Build history of the part. All positions in model axes, mm. Round coordinates to 2 decimals unless told otherwise and drop trailing zeros. Write each loop counter-clockwise with the first axis right and the second up, starting at its lowest first coordinate (ties: lowest second). Pieces come first, ordered by that corner, then holes.
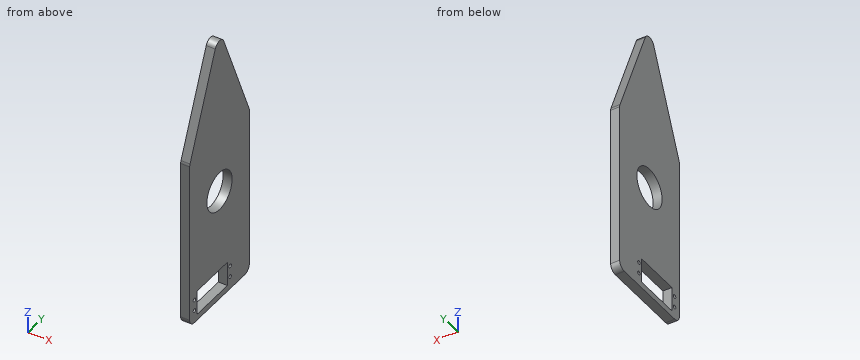
from build123d import *

# Parameters (mm, degrees)
SKETCH1_R                             = 17.4625
BOSS_EXTRUDE2_DEPTH                   = 4.0005
FILLET1_R                             = 6.35
TAP_DRILL_FOR_M4X0_7_TAP1_D           = 3.3
TAP_DRILL_FOR_M4X0_7_TAP1_CSINK_D     = 3.35
TAP_DRILL_FOR_M4X0_7_TAP1_CSINK_ANGLE = 90
SKETCH5_W                             = 42
SKETCH5_H                             = 22
CUT_EXTRUDE1_DEPTH                    = 148.97697313


with BuildPart() as part:
    # Sketch1 → Boss-Extrude2 (new, symmetric)
    with BuildSketch(Plane.YZ):
        Polygon((-41.275, 50.8), (-41.275, -101.6), (41.275, -101.6), (41.275, 50.8), (0, 152.4), align=None)
        with Locations(Location((0, 0, 0), (0, 0, 270))):
            Circle(SKETCH1_R, mode=Mode.SUBTRACT)
    extrude(amount=BOSS_EXTRUDE2_DEPTH, both=True)

    # Fillet1
    fillet1_edges = [part.edges().sort_by_distance(p)[0] for p in [
        (0, 0, 152.4),
        (0, 41.275, 50.8),
        (0, 41.275, -101.6),
        (0, -41.275, -101.6),
        (0, -41.275, 50.8),
    ]]
    fillet(fillet1_edges, radius=FILLET1_R)

    # Tap Drill for M4x0.7 Tap1 (through all)
    with Locations(Plane.YZ.offset(4.0005)):
        with Locations((-34.75, -80.25), (-34.75, -90.25), (14.75, -80.25), (14.75, -90.25)):
            CounterSinkHole(TAP_DRILL_FOR_M4X0_7_TAP1_D / 2, TAP_DRILL_FOR_M4X0_7_TAP1_CSINK_D / 2, counter_sink_angle=TAP_DRILL_FOR_M4X0_7_TAP1_CSINK_ANGLE)

    # Sketch5 → Cut-Extrude1 (cut, through all)
    with BuildSketch(Plane.YZ.offset(4.0005)):
        with Locations((-10, -85.25)):
            Rectangle(SKETCH5_W, SKETCH5_H)
    extrude(amount=-CUT_EXTRUDE1_DEPTH, mode=Mode.SUBTRACT)


solid = part.part
1) Wall check: L1, parallel to Y at x = 2.5, z = -80.25 (3 decimals); L2, parallel to Z at x = -3.25, y = -0.5; L3, parallel to Z at x = -2, y = 5. Give the ranges that are in metal, low to high.
Results:
L1: y = -41.275 to -36.4, -33.1 to -31, 11 to 13.1, 16.4 to 41.275
L2: z = -101.6 to -96.25, -74.25 to -17.46, 17.46 to 141.86
L3: z = -101.6 to -96.25, -74.25 to -16.73, 16.73 to 139.44
2) Slice it at A-A (x = -2.5). Count the separate pieces of the cut face and the enclosed holes in it, plus the area to 3 significant figures.
Results:
separate pieces: 1
enclosed holes: 6
area: 14,800 mm2
3) Pin check, flat tips, straight feed: pin 1 Ø1 at (x, y) = (-1, 31.5) entering from +Z; pin 2 Ø4 at (x, y) = (-0.5, -19.5) entering from +Z; pin 3 Ø2.5 at (y, z) = (-34.75, -90.25) entering from -X; pin 4 Ø2 at (x, y) = (1, -4) entering from +Z. Stop position of each tip, or through.
Results:
pin 1: stops at z = 76.09
pin 2: stops at z = 109.32
pin 3: passes through
pin 4: stops at z = 141.13
4) Slice it at B-B (z = 0). Write the cut outline in (x, y) (1 decimal).
Results:
outline: (-4, -41.3) - (4, -41.3) - (4, -17.5) - (-4, -17.5) - close; (-4, 17.5) - (4, 17.5) - (4, 41.3) - (-4, 41.3) - close
5) Slice it at D-D (y = 31). Write the cut outline in (x, z), plus the area to 3 significant figures.
Results:
outline: (-4, -101.6) - (4, -101.6) - (4, 76.09) - (-4, 76.09) - close
area: 1,420 mm2
6) Slice it at C-C (y = 0). Write the cut outline in (x, z).
Results:
outline: (-4, -101.6) - (4, -101.6) - (4, -96.25) - (-4, -96.25) - close; (-4, -74.25) - (4, -74.25) - (4, -17.46) - (-4, -17.46) - close; (-4, 17.46) - (4, 17.46) - (4, 141.88) - (-4, 141.88) - close
